Geometry: see drawing. Coordinates: mm, zero at the bounding-box minimum. A direction names the side the tool comes from. Give positions to 0.01 mm unless a question says otherwise; leave off trailing zeros. Write each loop counter-clockwise with the first axis right and the second up, starting at its lowest first coordinate (ties: lowest second). Pieces come first, ordered by that corner, then holes. Notation, with made-up numbers: (68, -13.75) -> (108, -13.75) arc R32 ccw to (108, 25.25) -> close; hole circle Ø7 at (33.5, 11). An arc over 180 degrees is marked (long way). Answer as a JSON object with one key per item and string values. Group by question number.
Item 1: Section query A-A on x = 17.25. Return the cut outline in (y, z), plus the area to 3 significant figures.
Item 2: First-contact query: pin 1 Ø2.5 at (y, z) = (15, 34.85) entering from -X; pin 2 Ø1 at (x, y) = (10.5, 11.5) entering from -Z. Flat tips, straight axial feed; report the tip coordinate or a pass-through.
Item 3: Section query D-D on z = 34.85. Return the cut outline in (x, y).
Item 4: Section query B-B on y = 15. Return the cut outline in (x, z).
Item 5: Access query for the marked faces 1, 2, 3 and 4. Directions: +Z, -Z, +X, -X, +Y, -Y. A direction counts if a zero-diameter tool reaches every point of the face in a straight line with its end or side. Return the directions, or none.
Item 6: Ray query, probe 1 along Y at (x, z) = (13, 17). Return the intervals inside material, ascending. Write a range as from..to.
Item 7: Pull-direction query (Z, two-part tool) for the marked faces 5, 6 and 7; classes: pulls with the +Z half, pulls with the -Z half, needs draft (parallel to the pull), parting line crosses it, or undercut.
Item 8: Section query C-C on z = 16.5. Return the cut outline in (x, y).
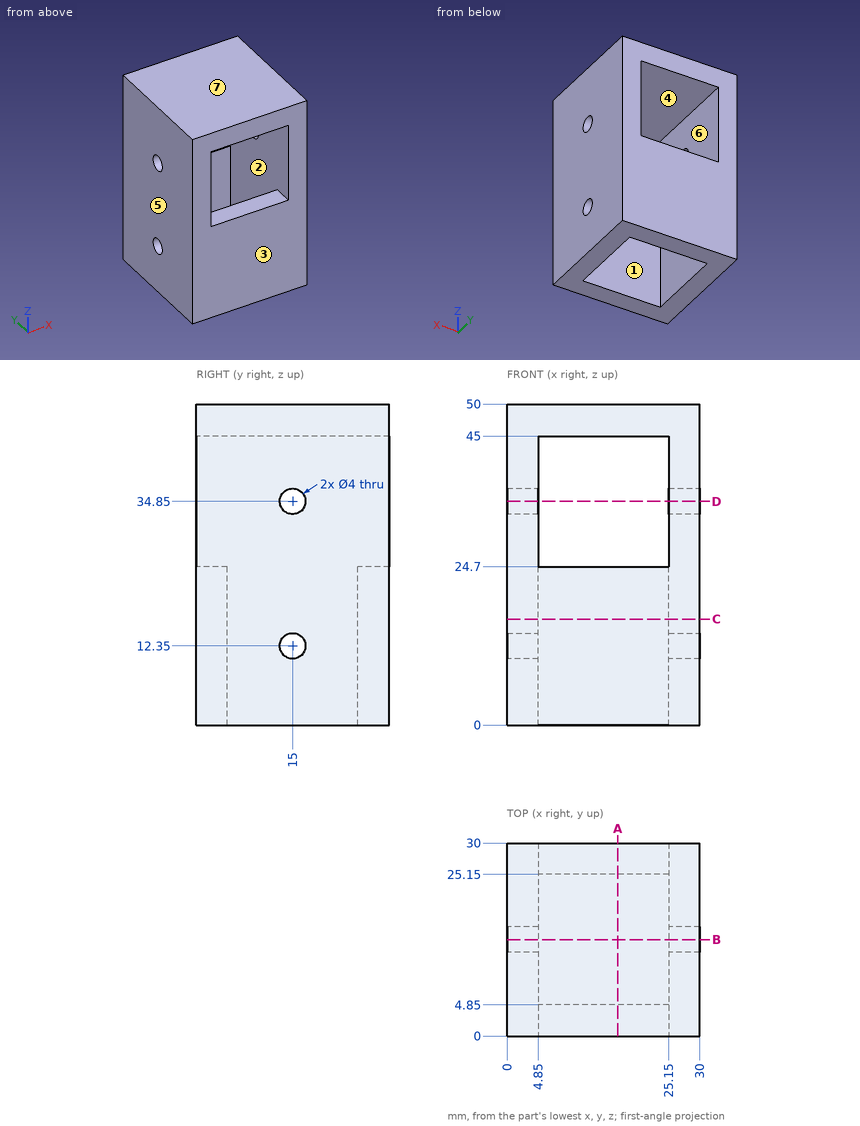
Worked answers:
{
 "1": {"outline": "(0, 0) -> (4.85, 0) -> (4.85, 24.7) -> (0, 24.7) -> close; (0, 45) -> (30, 45) -> (30, 50) -> (0, 50) -> close; (25.15, 0) -> (30, 0) -> (30, 24.7) -> (25.15, 24.7) -> close", "area": "390 mm^2"},
 "2": {"pin 1": "through", "pin 2": "z = 45"},
 "3": {"outline": "(0, 0) -> (4.85, 0) -> (4.85, 13) -> (0, 13) -> close; (0, 17) -> (4.85, 17) -> (4.85, 30) -> (0, 30) -> close; (25.15, 0) -> (30, 0) -> (30, 13) -> (25.15, 13) -> close; (25.15, 17) -> (30, 17) -> (30, 30) -> (25.15, 30) -> close"},
 "4": {"outline": "(0, 0) -> (4.85, 0) -> (4.85, 10.35) -> (0, 10.35) -> close; (0, 14.35) -> (4.85, 14.35) -> (4.85, 32.85) -> (0, 32.85) -> close; (0, 36.85) -> (4.85, 36.85) -> (4.85, 45) -> (25.15, 45) -> (25.15, 36.85) -> (30, 36.85) -> (30, 50) -> (0, 50) -> close; (25.15, 0) -> (30, 0) -> (30, 10.35) -> (25.15, 10.35) -> close; (25.15, 14.35) -> (30, 14.35) -> (30, 32.85) -> (25.15, 32.85) -> close"},
 "5": {"face 1": "-Z", "face 2": "none", "face 3": "+Z, -Z, +X, -X, -Y", "face 4": "+Y, -Y"},
 "6": {"probe 1": "0..4.85, 25.15..30"},
 "7": {"face 5": "needs draft", "face 6": "undercut", "face 7": "pulls with the +Z half"},
 "8": {"outline": "(0, 0) -> (30, 0) -> (30, 30) -> (0, 30) -> close; hole (4.85, 4.85) -> (25.15, 4.85) -> (25.15, 25.15) -> (4.85, 25.15) -> close"}
}
